Could you check a few things on this drawing? It's one solid part, dimensions in mm from its lowest x, y, z. Give positions to 0.01 mm unless a question says otherwise; leave off trailing zeros. Order: outer loops, then holes, each group sorted by start corner. A loop starts at its lowest first (then second) coordinate and runs counter-clockwise, first axis right, second up. Notation, with made-up numbers: M 52,77 L 69,77 A35 ccw 69,111 Z; hole C 46.5,75 d10. An arc over 180 degrees is marked long. Use one line per item in the form item = value.
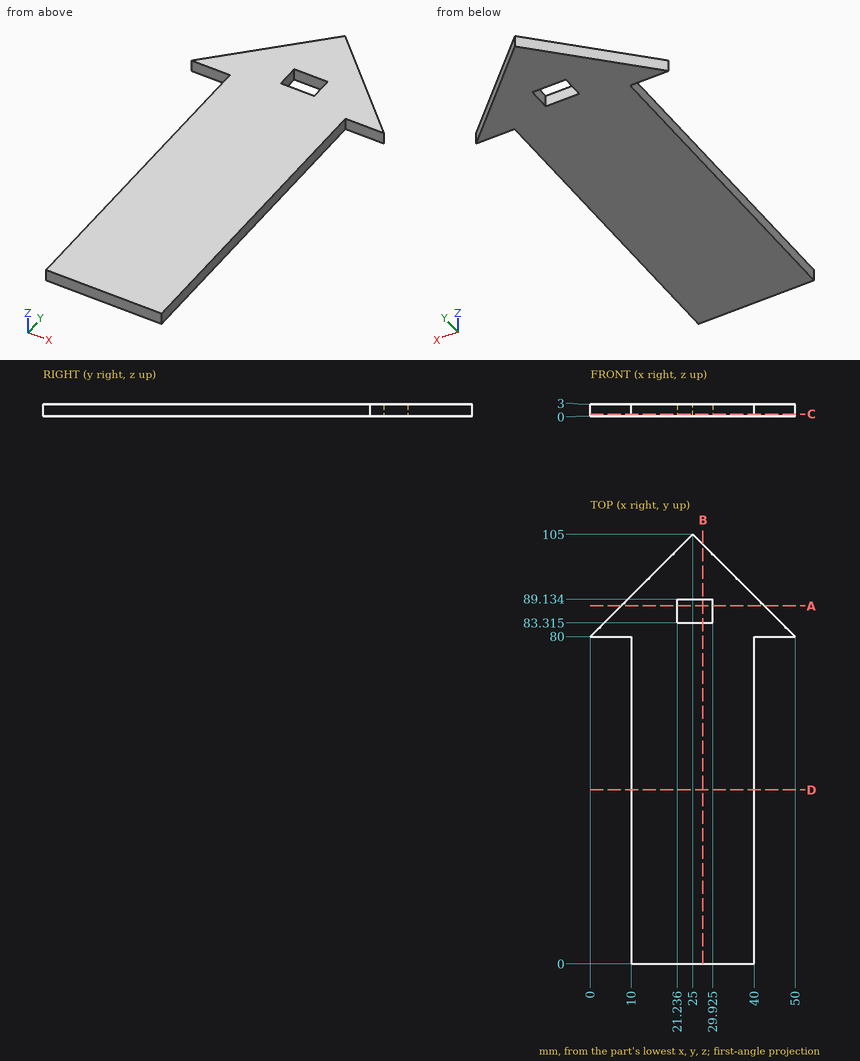
Q1. I want a section at C-C on z = 0.5. Write out the boundary of the cut face in (x, y) (1 decimal), then the cut area to 3 significant figures.
Found:
outline = M 0,80 L 10,80 L 10,0 L 40,0 L 40,80 L 50,80 L 25,105 Z; hole M 21.2,83.3 L 29.9,83.3 L 29.9,89.1 L 21.2,89.1 Z
area = 2,970 mm²
Q2. I want a section at D-D on y = 42.5. Write out the boundary of the cut face in (x, z).
Found:
outline = M 10,0 L 40,0 L 40,3 L 10,3 Z
Q3. I want a section at A-A on y = 87.5. Write out the boundary of the cut face in (x, z) (1 decimal).
Found:
outline = M 7.5,0 L 21.2,0 L 21.2,3 L 7.5,3 Z; M 29.9,0 L 42.5,0 L 42.5,3 L 29.9,3 Z
Q4. I need wall thicknesses on L1, parallel to X at y = 33, z = 2.7; L2, parallel to Y at x = 22.5, z = 1.85 (1 decimal); L3, parallel to Y at x = 23.5, z = 0.8 (1 decimal). Which ranges of each line are inside material? Lowest first, please.
Found:
L1 = 10 to 40
L2 = 0 to 83.3, 89.1 to 102.5
L3 = 0 to 83.3, 89.1 to 103.5
Q5. I'm going to push flat-ended pins straight in: pin 1 Ø0.9 at (y, z) = (85, 1) entering from -X; pin 2 Ø0.9 at (y, z) = (49, 1) entering from -X. Where does each tip first touch, or does it pass through?
Found:
pin_1 = 4.55
pin_2 = 10
Q6. I want a section at B-B on x = 27.5. Write out the boundary of the cut face in (y, z) (1 decimal), then the cut area to 3 significant figures.
Found:
outline = M 0,0 L 83.3,0 L 83.3,3 L 0,3 Z; M 89.1,0 L 102.5,0 L 102.5,3 L 89.1,3 Z
area = 290 mm²
